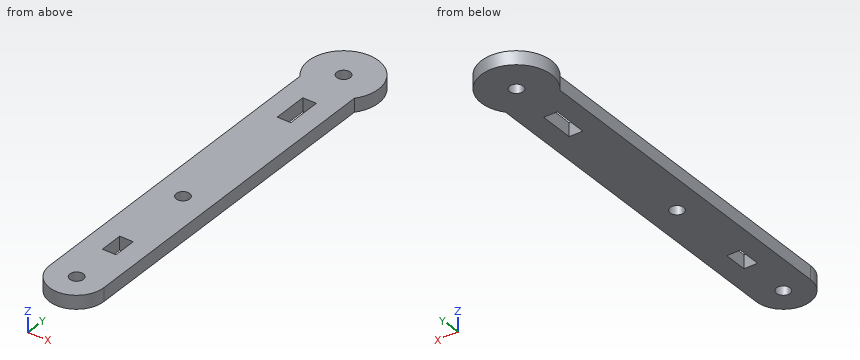
```python
from build123d import *

# Parameters (mm, degrees)
ESQUISSE1_W        = 3
ESQUISSE1_H        = 5.2
ESQUISSE1_R        = 1.5
ESQUISSE1_H_2      = 7.7
BOSS_EXTRU_1_DEPTH = 3


with BuildPart() as part:
    # Esquisse1 → Boss.-Extru.1 (new body)
    with BuildSketch(Plane.XY):
        with BuildLine():
            ThreePointArc((771.396898563, 207.86630439), (765.396898563, 220.521658607), (759.396898563, 207.86630439))
            Line((759.396898563, 207.86630439), (759.396898563, 132.443292949))
            ThreePointArc((759.396898563, 132.443292949), (765.396898563, 126.443292949), (771.396898563, 132.443292949))
            Line((771.396898563, 132.443292949), (771.396898563, 207.86630439))
        make_face()
        with Locations((765.396898563, 144.843292949)):
            Rectangle(ESQUISSE1_W, ESQUISSE1_H, mode=Mode.SUBTRACT)
        with Locations((765.396898563, 132.443292949)):
            Circle(ESQUISSE1_R, mode=Mode.SUBTRACT)
        with Locations((765.396898563, 164.443292949)):
            Circle(ESQUISSE1_R, mode=Mode.SUBTRACT)
        with Locations((765.396898563, 198.693292949)):
            Rectangle(ESQUISSE1_W, ESQUISSE1_H_2, mode=Mode.SUBTRACT)
        with Locations((765.396898563, 212.771658607)):
            Circle(ESQUISSE1_R, mode=Mode.SUBTRACT)
    extrude(amount=BOSS_EXTRU_1_DEPTH)


solid = part.part
```
The listing builds one solid part. Answer for the finished solid, in the listing's coordinates (mm). Coordinates: 2 decimals unless noted, no trailing zeros. Write each loop counter-clockwise with the first axis right and the second up, starting at its lowest first coordinate (ties: lowest second). Pieces come first, ordered by that corner, then holes. Notation, with made-up numbers: M -28,64 L 7,64 A16 cw 7,78 Z; hole C 64.25,57 d9. An arc over 180 degrees is marked long. Use a Markdown table: item, result. Add a question column.
1. Section B-B (y = 190.5) is taken. Give the vertices of the cut face in (x, z), plus the area to 3 significant figures.
2. Section A-A (z = 0.85) is taken. Give the vertices of the cut face in (x, y).
3. Section C-C (x = 770.5) is taken. Give the vertices of the cut face in (y, z).
4. Straight lines are drawn through the part: line 1 along X through (y, z) = (132.5, 2.35); line 2 along Y through (x, z) = (766.5, 1.2); line 3 along Y through (x, z) = (766.75, 1.9). For each, find the intervals that lie inside material, in ascending order. Write a range as [from, to].
5. Given P1, Ø1, axis at x = 760, z = 2.5, coming from the +Y side; P2, Ø1.5, axis at y = 180.5, z = 2, coming from the +X side; P3, Ø1, axis at y = 210.5, z = 1, coming from the -X side, each flat-ended and moving along its own axis, determine where each tip first touches the part or whether it passes through.
Data:
| question | item | result |
|---|---|---|
| 1 | outline | M 759.4,0 L 771.4,0 L 771.4,3 L 759.4,3 Z |
| 1 | area | 36.0 mm2 |
| 2 | outline | M 759.4,132.44 A6 ccw 771.4,132.44 L 771.4,207.87 A7.75 ccw long 759.4,207.87 Z; hole C 765.4,132.44 d3; hole M 763.9,142.24 L 766.9,142.24 L 766.9,147.44 L 763.9,147.44 Z; hole C 765.4,164.44 d3; hole M 763.9,194.84 L 766.9,194.84 L 766.9,202.54 L 763.9,202.54 Z; hole C 765.4,212.77 d3 |
| 3 | outline | M 129.29,0 L 218.6,0 L 218.6,3 L 129.29,3 Z |
| 4 | line 1 | x = [759.4, 763.9], [766.9, 771.4] |
| 4 | line 2 | y = [126.55, 131.43], [133.46, 142.24], [147.44, 163.43], [165.46, 194.84], [202.54, 211.76], [213.79, 220.44] |
| 4 | line 3 | y = [126.6, 131.8], [133.09, 142.24], [147.44, 163.8], [165.09, 194.84], [202.54, 212.12], [213.42, 220.4] |
| 5 | P1 | stops at y = 218.78 |
| 5 | P2 | stops at x = 771.4 |
| 5 | P3 | stops at x = 757.85 |
